CAD build for the part. Positions are in the model's coordinates, mm. Face numbers are marked on the shaded views. A direction names the side the tool comes from. Coordinates: 2 decimals unless noted, no trailing zeros. Order: outer loops, then holes, each group sorted by start corner. A loop starts at its lowest first (then second) coordinate and runs counter-clockwise, first axis right, second up.
Autodesk Inventor part; units mm, degrees
ref_plane "YZ Plane" through (0, 0, 0) normal (1, 0, 0) x (0, 1, 0)
ref_plane "XZ Plane" through (0, 0, 0) normal (0, 1, 0) x (-1, 0, 0)
ref_plane "XY Plane" through (0, 0, 0) normal (0, 0, 1) x (1, 0, 0)
sketch "Sketch1" plane through (0, 0, 0) normal (0, 0, 1) x (1, 0, 0)
  line L0 (-4.2, 0) -> (0.7, 0) construction
  line L1 (0, -3.05) -> (0, 18.3) construction
  line L2 (0, 5) -> (-3.5, 5)
  line L3 (-3.5, 5) -> (-3.5, 15.25)
  line L4 (-3.5, 15.25) -> (-1.5, 15.25)
  line L5 (-1.5, 15.25) -> (-1.5, 10.5)
  line L6 (-1.5, 10.5) -> (0, 10.5)
  line L7 (0, 10.5) -> (0, 5)
  point P0 (0, 0)
  dimension "d0" = 10
  dimension "d1" = 21
  dimension "d2" = 1.5
  dimension "d3" = 2
  dimension "d4" = 30.5
revolve "Revolution1" add sketch "Sketch1" angle 360 about axis through (-10, 0, 0) along (1, 0, 0)
sketch "Sketch2" plane through (-3.5, 0, 0) normal (-1, 0, 0) x (0, 0, 1)
  line L0 (0, -21.35) -> (0, 21.35)
  line L1 (-21.35, 0) -> (21.35, 0)
  point P0 (0, 0)
  point P1 (0, 13)
  dimension "d6" = 13
hole "Hole1" at (-3.5, 13, 0) direction (1, 0, 0) diameter 2.8 end through all
mirror "Mirror1" about plane through (0, 0, 0) normal (0, 1, 0) of "Hole1"
fillet "Fillet1" radius 0.2 2 edges at (0, -10.5, 0) (0, -5, 0)
properties part number "P120RondelleAppui" material "ABS Plastic"
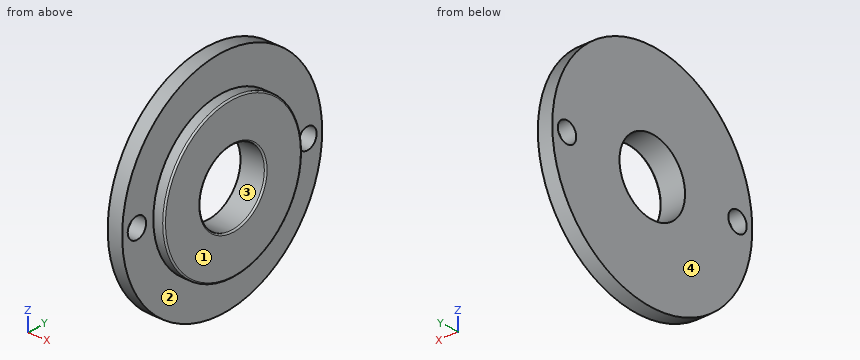
1) Drill centre lines: probe 1 along Z at (x, y) = (-0.9, 0); probe 2 along Z at (x, y) = (-1.7, 0); probe 3 along Y at (x, z) = (-2.9, 0.5). Where is each one in solid material? Low to high.
2) Slice it at A-A (z = 0). List the corners of the cut face in (x, y), plus the area to 3 significant figures.
3) Slice it at B-B (y = 0). List the corners of the cut face in (x, z), plus the area to 3 significant figures.
4) Two-plate mould, pull along Z, no slides. Class the marked faces 3 and 4: released by +Z, released by -Z, zero draft, split by the parting line, or undercut.
5) Pin check, flat tips, straight feed: P1, Ø4.5, axis at y = 13, z = 0, coming from the +X side; P2, Ø1, axis at x = -2, z = 6.5, coming from the +Y side. Stop position of each tip, or through.
6) Slice it at C-C (x = -2.6). List the corners of the cut face in (y, z).
7) Which spindle directions (+Z, -Z, +X, -X, +Y, -Y) get a long thin tool onto all of the face, cutting with end or side? Do the marked faces 1 and 2. Say none if no direction does.
8) Slice it at D-D (y = -13). List the corners of the cut face in (x, z).
Worked out:
1. probe 1: z = -10.5 to -5, 5 to 10.5
1. probe 2: z = -15.25 to -5, 5 to 15.25
1. probe 3: y = -15.24 to -14.31, -11.69 to -4.97, 4.97 to 11.69, 14.31 to 15.24
2. outline: (-3.5, -15.25) - (-1.5, -15.25) - (-1.5, -14.4) - (-3.5, -14.4) - close; (-3.5, -11.6) - (-1.5, -11.6) - (-1.5, -10.5) - (-0.2, -10.5) arc R0.2 ccw to (0, -10.3) - (0, -5.2) arc R0.2 ccw to (-0.2, -5) - (-3.5, -5) - close; (-3.5, 5) - (-0.2, 5) arc R0.2 ccw to (0, 5.2) - (0, 10.3) arc R0.2 ccw to (-0.2, 10.5) - (-1.5, 10.5) - (-1.5, 11.6) - (-3.5, 11.6) - close; (-3.5, 14.4) - (-1.5, 14.4) - (-1.5, 15.25) - (-3.5, 15.25) - close
2. area: 46.3 mm2
3. outline: (-3.5, -15.25) - (-1.5, -15.25) - (-1.5, -10.5) - (-0.2, -10.5) arc R0.2 ccw to (0, -10.3) - (0, -5.2) arc R0.2 ccw to (-0.2, -5) - (-3.5, -5) - close; (-3.5, 5) - (-0.2, 5) arc R0.2 ccw to (0, 5.2) - (0, 10.3) arc R0.2 ccw to (-0.2, 10.5) - (-1.5, 10.5) - (-1.5, 15.25) - (-3.5, 15.25) - close
3. area: 57.5 mm2
4. face 3: undercut
4. face 4: zero draft
5. P1: stops at x = -1.5
5. P2: stops at y = 14.02
6. outline: circle Ø30.5 at (0, 0); hole circle Ø2.8 at (-13, 0); hole circle Ø10 at (0, 0); hole circle Ø2.8 at (13, 0)
7. face 1: +Z, -Z, +X, +Y, -Y
7. face 2: +X
8. outline: (-3.5, -7.97) - (-1.5, -7.97) - (-1.5, -1.4) - (-3.5, -1.4) - close; (-3.5, 1.4) - (-1.5, 1.4) - (-1.5, 7.97) - (-3.5, 7.97) - close
